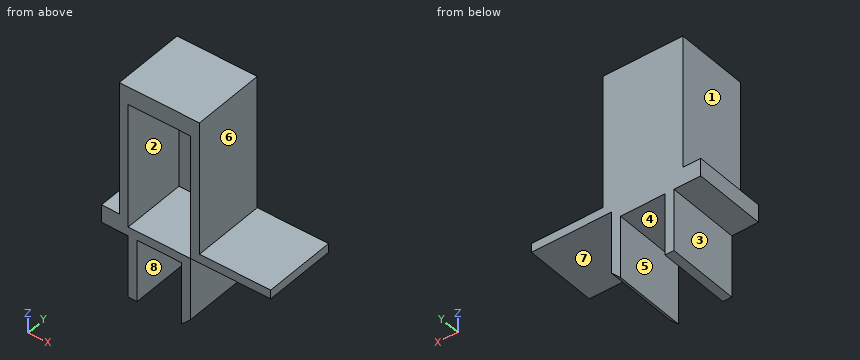
```python
from build123d import *

# Parameters (mm, degrees)
SKETCH011_W      = 7
SKETCH011_H      = 14
EXTRUDE012_DEPTH = 10
EXTRUDE_DEPTH    = 8.2


with BuildPart() as extrude012:
    # Sketch011 → Extrude012 (new body)
    with BuildSketch(Plane.XZ.offset(4.5)):
        with Locations((0, 31)):
            Rectangle(SKETCH011_W, SKETCH011_H)
    extrude(amount=EXTRUDE012_DEPTH)


with BuildPart() as extrude012_1:
    # Extrude012 placement: moved
    add(extrude012.part.moved(Location((0, 7.6, 0))))


with BuildPart() as button001:
    # Sketch → Extrude (new body)
    with BuildSketch(Plane.XZ.offset(4.5)):
        Polygon((-6.5, 23), (-3.5, 23), (-3.5, 16), (-2.5, 16), (-2.5, 23), (2.5, 23), (2.5, 16), (3.5, 17), (3.5, 24), (12.5, 24), (12.5, 25), (4.5, 25), (4.5, 40), (-4.5, 40), (-4.5, 25), (-6.5, 25), align=None)
    extrude(amount=-EXTRUDE_DEPTH)


with BuildPart() as button001_1:
    # Extrude placement: moved
    add(button001.part.moved(Location((0, 0.4, 0))))

    # Cut001: cut Extrude012
    add(extrude012_1.part, mode=Mode.SUBTRACT)


solid = button001_1.part
```
Geometry check sheet. Reference: the model listing, model coordinates, mm. Face numbers are marked on the shaded views. A direction names the side the tool comes from. Round coordinates to 2 decimals unless told otherwise and drop trailing zeros. Order: outer loops, then holes, each group sorted by start corner. A loop starts at its lowest first (then second) coordinate and runs counter-clockwise, first axis right, second up. Notation, with made-up numbers: (-34, -12.75) - (-24, -12.75) arc R21 ccw to (-24, 0.25) - close; hole circle Ø1 at (-14.75, 71). An arc over 180 degrees is marked (long way). Use a Markdown table: item, result. Add a question column.
1) Section check B-B (y = 3.5). Record the cut outline in (x, z).
2) Gauge pin test, flat ends, axial feed: P1, Ø1.5, axis at y = -2.5, z = 37, coming from the +X side; P2, Ø3.5, axis at x = 0, z = 34.5, coming from the -Y side; P3, Ø4, axis at y = -0.5, z = 25.5, coming from the +X side; P4, Ø2, axis at y = 1.5, z = 21.5, coming from the +X side. Record the tip position at first contact, or that the pin passes through.
3) Thickness scan on line 1 along X through (y, z) = (-2.25, 36.25); line 2 along X through (y, z) = (-1, 21.5); line 3 along Z through (x, y) = (1.25, -0.5). Record the ranges inside material, lowest first.
4) Mould release check, pull along X, two halves, no side actions. Record for the marked faces 5, 6, 7 and 8: released by +X, released by -X, zero draft, split by the parting line, or undercut.
5) Section check C-C (x = 1.75). Record the cut outline in (y, z).
6) Section check A-A (z = 22.5). Record the cut outline in (x, y), then the cut area to 3 significant figures.
7) Set-up check for the marked faces 1, 2, 3 and 4: record each of +Z, -Z, +X, -X, +Y, -Y from which the full face is reachable in a straight line by a thin tool's end or side.
Established:
| question | item | result |
|---|---|---|
| 1 | outline | (-6.5, 23) - (-3.5, 23) - (-3.5, 16) - (-2.5, 16) - (-2.5, 23) - (2.5, 23) - (2.5, 16) - (3.5, 17) - (3.5, 24) - (12.5, 24) - (12.5, 25) - (4.5, 25) - (4.5, 40) - (-4.5, 40) - (-4.5, 25) - (-6.5, 25) - close |
| 2 | P1 | x = 4.5 |
| 2 | P2 | y = 3.1 |
| 2 | P3 | x = 12.5 |
| 2 | P4 | x = 3.5 |
| 3 | line 1 | -4.5 to -3.5, 3.5 to 4.5 |
| 3 | line 2 | -3.5 to -2.5, 2.5 to 3.5 |
| 3 | line 3 | 23 to 24, 38 to 40 |
| 4 | face 5 | undercut |
| 4 | face 6 | released by +X |
| 4 | face 7 | zero draft |
| 4 | face 8 | undercut |
| 5 | outline | (-4.1, 23) - (4.1, 23) - (4.1, 40) - (-4.1, 40) - (-4.1, 38) - (3.1, 38) - (3.1, 24) - (-4.1, 24) - close |
| 6 | outline | (-3.5, -4.1) - (-2.5, -4.1) - (-2.5, 4.1) - (-3.5, 4.1) - close; (2.5, -4.1) - (3.5, -4.1) - (3.5, 4.1) - (2.5, 4.1) - close |
| 6 | area | 16.4 mm2 |
| 7 | face 1 | +Z, -X, +Y, -Y |
| 7 | face 2 | -Y |
| 7 | face 3 | -Z, -X, +Y, -Y |
| 7 | face 4 | -Z, +Y, -Y |
